Source: three-view drawing plus pictorial views. Frame: mm from the lowest corner of the part. A direction names the side the tool comes from. Give positions to 0.01 mm unless a question says otherwise; leave off trailing zeros. Order: outer loops, then holes, each group sorted by start corner. A loop starts at its lowest first (then second) coordinate and runs counter-clockwise, first axis right, second up. Notation, with made-up numbers: (55, 80.25) -> (75, 80.25) arc R27 ccw to (75, 105.25) -> close; hole circle Ø5 at (62, 34). An arc over 180 degrees is marked (long way). Answer in a Markdown table with one row per item.
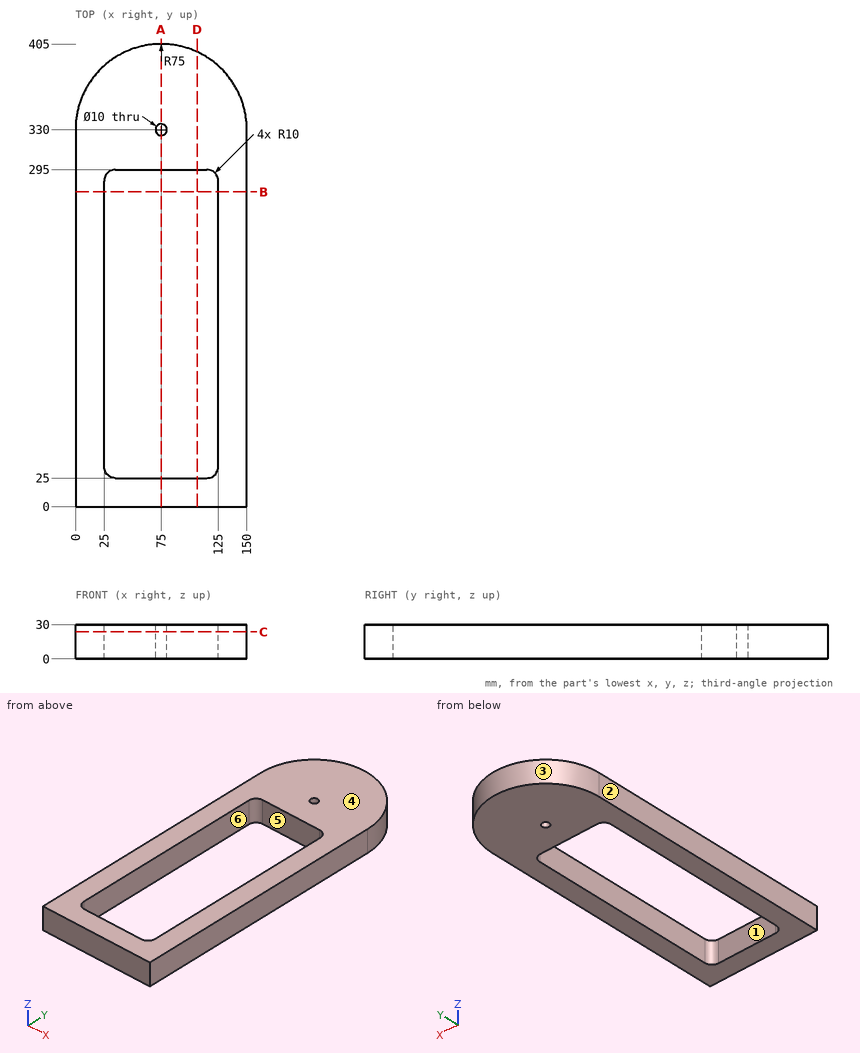
(1) Section query D-D (x = 106.5). Return the cut outline in (y, z), plus the area to 3 significant figures.
A:
| item | result |
|---|---|
| outline | (0, 0) -> (25, 0) -> (25, 30) -> (0, 30) -> close; (295, 0) -> (398.06, 0) -> (398.06, 30) -> (295, 30) -> close |
| area | 3,840 mm^2 |
(2) Pull-direction query (X, two-part tool) for the marked faces 3, 4, 5 and 6; classes: +X half, -X half, draft (parallel to the pull), parting line (faces both ways), or undercut.
A:
| item | result |
|---|---|
| face 3 | parting line |
| face 4 | draft |
| face 5 | undercut |
| face 6 | undercut |
(3) Section query A-A (x = 75). Return the cut outline in (y, z).
A:
| item | result |
|---|---|
| outline | (0, 0) -> (25, 0) -> (25, 30) -> (0, 30) -> close; (295, 0) -> (325, 0) -> (325, 30) -> (295, 30) -> close; (335, 0) -> (405, 0) -> (405, 30) -> (335, 30) -> close |
(4) Section query B-B (y = 275.5). Return the cut outline in (x, z).
A:
| item | result |
|---|---|
| outline | (0, 0) -> (25, 0) -> (25, 30) -> (0, 30) -> close; (125, 0) -> (150, 0) -> (150, 30) -> (125, 30) -> close |
(5) First-contact query: pin 1 Ø10 at (x, z) = (22.5, 12.5) entering from +Y; pin 2 Ø1 at (x, z) = (73, 4) entering from +Y (3 decimals). Flat tips, straight axial feed; report the tip coordinate or a pass-through.
A:
| item | result |
|---|---|
| pin 1 | stops at y = 388.04 |
| pin 2 | stops at y = 404.985 |
(6) Ray query, probe 1 along Y at (x, z) = (75, 7.75); probe 2 along X at (y, z) = (330, 9.25); probe 3 along X at (y, z) = (133.5, 23.25). Return the intervals inside material, ascending.
A:
| item | result |
|---|---|
| probe 1 | y = 0 to 25, 295 to 325, 335 to 405 |
| probe 2 | x = 0 to 70, 80 to 150 |
| probe 3 | x = 0 to 25, 125 to 150 |
(7) Access query for the marked faces 1 and 2. Directions: +Z, -Z, +X, -X, +Y, -Y. A direction counts if a zero-diameter tool reaches every point of the face in a straight line with its end or side. Return the directions, or none.
A:
| item | result |
|---|---|
| face 1 | +Z, -Z |
| face 2 | +Z, -Z, -X, +Y, -Y |
(8) Section query C-C (z = 23.75). Return the cut outline in (x, y), plus the area to 3 significant figures.
A:
| item | result |
|---|---|
| outline | (0, 0) -> (150, 0) -> (150, 330) arc R75 ccw to (0, 330) -> close; hole (25, 35) arc R10 ccw to (35, 25) -> (115, 25) arc R10 ccw to (125, 35) -> (125, 285) arc R10 ccw to (115, 295) -> (35, 295) arc R10 ccw to (25, 285) -> close; hole circle Ø10 at (75, 330) |
| area | 31,300 mm^2 |
